Read the model definition and answer for the solid it produces. Units are mm, in the model's axes. A direction names the side the tool comes from. Coordinates: 2 decimals unless noted, no trailing zeros. Loops run counter-clockwise (first coordinate to the right, second up) from the corner with the lowest first, then second, coordinate; pieces in that order, holes last. Notation, with made-up numbers: (14, 29) -> (54, 29) arc R7 ccw to (54, 36) -> close; hole circle Ø8 at (19.5, 54.5). An arc over 180 degrees is marked (long way). Answer as a JSON object with one key per item and string values. Group by question number.
1) Consider probe 1 along X at (y, z) = (12, -15.5); probe 2 along Z at (x, y) = (1, 4.75); probe 3 along X at (y, z) = (10, -34.95). Determine where each line is inside the solid, lowest interval first. Write a range as [from, to].
2) Section A-A, the plane y = 5 is taken. Give the vertices of the cut face in (x, z).
3) Flat-ended cylindrical pins translate along their axes: P1, Ø5.5, axis at y = 9, z = -39.5, coming from the -X side; P2, Ø2, axis at y = 8.5, z = -43, coming from the +X side; P3, Ø2, axis at x = 2, z = -44, coming from the -Y side. Find the tip coordinate at first contact, or state that the pin passes through.
4) Section D-D, the plane y = 3 is taken. Give the vertices of the cut face in (x, z), plus the area to 3 significant figures.
5) Section C-C, the plane z = -36.5 is taken. Give the vertices of the cut face in (x, y), plus the area to 3 significant figures.
6) Determine the mould class of faces 5 (the face through (0, 2, -27)), 6 (the face through (-0.1, 3.3, -21.2)), 7 (the face through (-4.5, 9, -19)), 8 (the face through (0.098, 10.744, -3.186)) for opening direction Y: released by +Y, released by -Y, zero draft, split by the parting line, or undercut.
7) Which of the six approach directions +Z, -Z, +X, -X, +Y, -Y give full straight-line access (tool end or side, diameter ignored) to faces 1 (the face through (-0.715, 3.225, -31.116)), 2 (the face through (0.063, 5.205, -7.376)), 3 (the face through (3, 10, -42)), 4 (the face through (-5, 10, -42))?
8) Section B-B, the plane x = -2.5 is taken. Give the vertices of the cut face in (y, z).
Autodesk Inventor part; units mm, degrees
ref_plane "Work Plane1" through (4.5, 0, 0) normal (1, 0, 0) x (0, 0, -1)
ref_plane "YZ Plane" through (0, 0, 0) normal (1, 0, 0) x (0, 1, 0)
ref_plane "XZ Plane" through (0, 0, 0) normal (0, 1, 0) x (-1, 0, 0)
sketch "Sketch2" plane through (0, 0, 0) normal (1, 0, 0) x (0, 1, 0)
  line L0 (0, 0) -> (0, -5)
  line L1 (13, 0) -> (13, -18)
  arc A0 (13, 0) -> (0, 0) centre (6.5, 0) ccw
  line L2 (-3.1385, 0) -> (18.8309, 0)
  line L3 (0, -54.8723) -> (0, 16.7287)
  line L4 (0, -5) -> (6.5, -11.5)
  line L5 (0, -5) -> (9.1924, -5) construction
  line L6 (6.5, -11.5) -> (6.5, -18)
  line L7 (6.5, -18) -> (0, -24.5)
  line L8 (6.5, -18) -> (15.6924, -18) construction
  line L9 (0, -24.5) -> (0, -29.5)
  line L10 (0, -29.5) -> (6.5, -36)
  line L11 (0, -29.5) -> (9.1924, -29.5) construction
  line L12 (13, -18) -> (13, -36)
  line L13 (13, -36) -> (13, -42.5)
  arc A1 (6.5, -36) -> (13, -42.5) centre (11.1419, -37.8581) ccw
  circle A2 centre (9.75, -40) radius 1.625
  dimension "d3" = 18
  dimension "d4" = 13
  dimension "d9" = 45
  dimension "d10" = 6.5
  dimension "d11" = 5
  dimension "d12" = 6.5
  dimension "d13" = 135
  dimension "d14" = 6.5
  dimension "d15" = 5
  dimension "d16" = 45
  dimension "d17" = 6.5
  dimension "d18" = 18
  dimension "d19" = 6.5
  dimension "d20" = 5
  dimension "d21" = 3.25
  dimension "d22" = 3.25
  dimension "d23" = 2.5
extrude "Extrusion1" add sketch "Sketch2" along normal mid plane 13 contours L2 L1 L12 L13 A1 L10 L3 L7 L6 L4 L0 | A0 L2
sketch "Sketch3" plane through (-6.5, 13, 0) normal (0, 1, 0) x (1, 0, 0)
  line L0 (0, 36) -> (13, 36)
  line L1 (0, 43) -> (1.5, 43)
  line L2 (1.5, 43) -> (1.5, 36)
  line L3 (1.5, 36) -> (0, 36)
  line L4 (0, 36) -> (0, 43)
  line L5 (0, 0) -> (0, 42.5)
  line L6 (3.5, 43) -> (7.5, 43)
  line L7 (7.5, 43) -> (7.5, 36)
  line L8 (7.5, 36) -> (3.5, 36)
  line L9 (3.5, 36) -> (3.5, 43)
  line L10 (9.5, 43) -> (13, 43)
  line L11 (13, 43) -> (13, 36)
  line L12 (13, 36) -> (9.5, 36)
  line L13 (9.5, 36) -> (9.5, 43)
  line L14 (13, 42.5) -> (13, 0)
  point P0 (6.5, 0)
  dimension "d47" = 1.5
  dimension "d48" = 7
  dimension "d49" = 4
  dimension "d50" = 7
  dimension "d51" = 2
  dimension "d52" = 7
  dimension "d53" = 2
extrude "Extrusion2" cut sketch "Sketch3" against normal blind 13
ref_plane "Work Plane1" through (4.5, 0, 0) normal (1, 0, 0) x (0, 0, -1)
sketch "Sketch4" plane through (4.5, 0, 0) normal (1, 0, 0) x (0, 0, -1)
  arc A0 (0, 13) -> (0, 0) centre (0, 6.5) ccw
  line L0 (0, 13) -> (36, 13)
  line L1 (36, 13) -> (36, 6.5)
  line L2 (36, 6.5) -> (29.5, 0)
  line L3 (29.5, 0) -> (24.5, 0)
  line L4 (24.5, 0) -> (18, 6.5)
  line L5 (36, 13) -> (36, 6.5)
  line L6 (36, 6.5) -> (29.5, 0)
  line L7 (29.5, 0) -> (24.5, 0)
  line L8 (24.5, 0) -> (18, 6.5)
  line L9 (18, 6.5) -> (11.5, 6.5)
  line L10 (11.5, 6.5) -> (5, 0)
  line L11 (5, 0) -> (0, 0)
  arc A1 (0, 13) -> (0, 0) centre (0, 6.5) ccw
  line L12 (0, 13) -> (36, 13)
  line L13 (0, 13) -> (0, 2)
  line L14 (0, 2) -> (2.1716, 2)
  line L15 (4.1716, 2) -> (10.6716, 8.5)
  line L16 (4.1716, 2) -> (13.364, 2) construction
  line L17 (34, 13) -> (34, 7.3284)
  line L18 (34, 7.3284) -> (28.6716, 2)
  line L19 (34, 7.3284) -> (41.5355, 7.3284) construction
  line L20 (28.6716, 2) -> (25.3284, 2)
  line L21 (25.3284, 2) -> (18.8284, 8.5)
  line L22 (25.3284, 2) -> (34.5208, 2) construction
  line L23 (18.8284, 8.5) -> (10.6716, 8.5)
  line L24 (4.1716, 2) -> (4.1716, 13)
  line L25 (2.1716, 2) -> (2.1716, 13)
  line L26 (0, 13) -> (2.1716, 13)
  line L27 (4.1716, 13) -> (34, 13)
  dimension "d57" = 11
  dimension "d58" = 2
  dimension "d59" = 45
  dimension "d60" = 2
  dimension "d62" = 2
  dimension "d63" = 2
  dimension "d64" = 135
  dimension "d65" = 2
  dimension "d66" = 2
  dimension "d67" = 135
  dimension "d94" = 2
  dimension "d95" = 2
extrude "Extrusion3" cut sketch "Sketch4" against normal blind 9 contours L0 L25 L14 L13 | L0 L17 L18 L20 L21 L23 L15 L24
sketch "Sketch5" plane through (4.5, 2, -4.1716) normal (0, 0, -1) x (-1, 0, 0)
  line L0 (0, 11) -> (0, 0)
  line L1 (9, 0) -> (9, 11)
  line L2 (0, 11) -> (0, 0)
  line L3 (0, 0) -> (9, 0)
  line L4 (9, 0) -> (9, 11)
  line L5 (0, 11) -> (9, 11)
  circle A0 centre (4.5, 8) radius 0.75
  circle A1 centre (4.5, 3) radius 0.75
  point P0 (4.5, -2)
  dimension "d72" = 1.5
  dimension "d73" = 4.5
  dimension "d74" = 3
  dimension "d75" = 1.5
  dimension "d76" = 3
  dimension "d77" = 4.5
extrude "Extrusion4" cut sketch "Sketch5" against normal blind 2 contours A0 | A1
sketch "Sketch6" plane through (1, 13, -36) normal (0, 0, -1) x (-1, 0, 0)
  line L0 (1, -15.6) -> (1, 2.6)
  line L1 (10.1, -13) -> (-8.1, -13)
  circle A0 centre (1, -3) radius 0.75
  line L2 (0, 0) -> (4, 0)
  circle A1 centre (1, -10) radius 0.75
  point P0 (1, -13)
  dimension "d80" = 1.5
  dimension "d81" = 3
  dimension "d82" = 1.5
  dimension "d83" = 3
extrude "Extrusion5" cut sketch "Sketch6" against normal blind 9
sketch "Sketch7" plane through (3, 13, -36) normal (1, 0, 0) x (0, 0, -1)
  line L0 (6.5, 0) -> (0, 0)
  line L1 (6.5, 0) -> (11.5, 0)
  line L2 (11.5, 0) -> (11.5, -2)
  line L3 (11.5, -2) -> (6.5, -2)
  line L4 (6.5, -2) -> (6.5, 0)
  point P0 (-36, -13)
  dimension "d86" = 5
  dimension "d87" = 2
extrude "Extrusion6" add sketch "Sketch7" against normal blind 2
sketch "Sketch8" plane through (-5, 13, -42.5) normal (-1, 0, 0) x (0, 0, 1)
  line L0 (0, 0) -> (6.5, 0)
  line L1 (-5, -2) -> (0, -2)
  line L2 (0, -2) -> (0, 0)
  line L3 (0, 0) -> (-5, 0)
  line L4 (-5, 0) -> (-5, -2)
  point P0 (42.5, -13)
  dimension "d90" = 5
  dimension "d91" = 2
extrude "Extrusion7" add sketch "Sketch8" against normal blind 2
properties part number "index"
Determined:
{
 "1": {"probe 1": "[-6.5, -4.5], [4.5, 6.5]", "probe 2": "[-34.25, -31.42], [-22.58, -19.75], [-9.75, -6.92], [-4.17, -2.17], [0, 6.26]", "probe 3": "[-6.5, -0.75], [0.75, 6.5]"},
 "2": {"outline": "(-6.5, -34.5) -> (6.5, -34.5) -> (6.5, -19.5) -> (-6.5, -19.5) -> close; (-6.5, -10) -> (6.5, -10) -> (6.5, 6.32) -> (-6.5, 6.32) -> close; hole (-4.5, -31.67) -> (4.5, -31.67) -> (4.5, -22.33) -> (-4.5, -22.33) -> close; hole (-4.5, -7.17) -> (4.5, -7.17) -> (4.5, -4.17) -> (0.75, -4.17) -> (0.75, -2.17) -> (4.5, -2.17) -> (4.5, 0) -> (-4.5, 0) -> (-4.5, -2.17) -> (-0.75, -2.17) -> (-0.75, -4.17) -> (-4.5, -4.17) -> close"},
 "3": {"P1": "x = -5", "P2": "x = 3", "P3": "y = 11"},
 "4": {"outline": "(-6.5, -32.5) -> (-0.75, -32.5) -> (-0.75, -29.67) -> (-4.5, -29.67) -> (-4.5, -24.33) -> (4.5, -24.33) -> (4.5, -29.67) -> (0.75, -29.67) -> (0.75, -32.5) -> (6.5, -32.5) -> (6.5, -21.5) -> (-6.5, -21.5) -> close; (-6.5, -8) -> (6.5, -8) -> (6.5, 5.48) -> (-6.5, 5.48) -> close; hole (-4.5, -5.17) -> (4.5, -5.17) -> (4.5, -4.17) -> (-4.5, -4.17) -> close; hole (-4.5, -2.17) -> (4.5, -2.17) -> (4.5, 0) -> (-4.5, 0) -> close", "area": "237 mm²"},
 "5": {"outline": "(-5, 6.33) -> (-3, 6.33) -> (-3, 13) -> (-5, 13) -> close; (1, 6.33) -> (3, 6.33) -> (3, 13) -> (1, 13) -> close", "area": "26.7 mm²"},
 "6": {"face 5": "released by +Y", "face 6": "released by -Y", "face 7": "zero draft", "face 8": "undercut"},
 "7": {"face 1": "-Z", "face 2": "+Y", "face 3": "-Z, +X, +Y, -Y", "face 4": "-Z, -X, +Y, -Y"},
 "8": {"outline": "(0, -29.5) -> (6.5, -36) -> (13, -36) -> (13, -34) -> (7.33, -34) -> (2, -28.67) -> (2, -25.33) -> (8.5, -18.83) -> (8.5, -10.67) -> (2, -4.17) -> (13, -4.17) -> (13, -2.17) -> (2, -2.17) -> (2, 0) -> (13, 0) arc R6.5 ccw to (0, 0) -> (0, -5) -> (6.5, -11.5) -> (6.5, -18) -> (0, -24.5) -> close"}
}
